Geometry check sheet. Reference: drawing and pictorial views, mm from the part's lowest x, y, z. A direction names the side the tool comes from. Round coordinates to 2 decimals unless told otherwise and drop trailing zeros. Loops run counter-clockwise (first coordinate to the right, second up) from the corner with the lowest first, then second, coordinate; pieces in that order, holes last. Notation, with made-up numbers: (46.25, 82.5) -> (58.25, 82.5) arc R12 ccw to (58.25, 101.5) -> close; hole circle Ø11 at (61.25, -7.75). An arc over 180 degrees is marked (long way). Use one line per item in the form item = value.
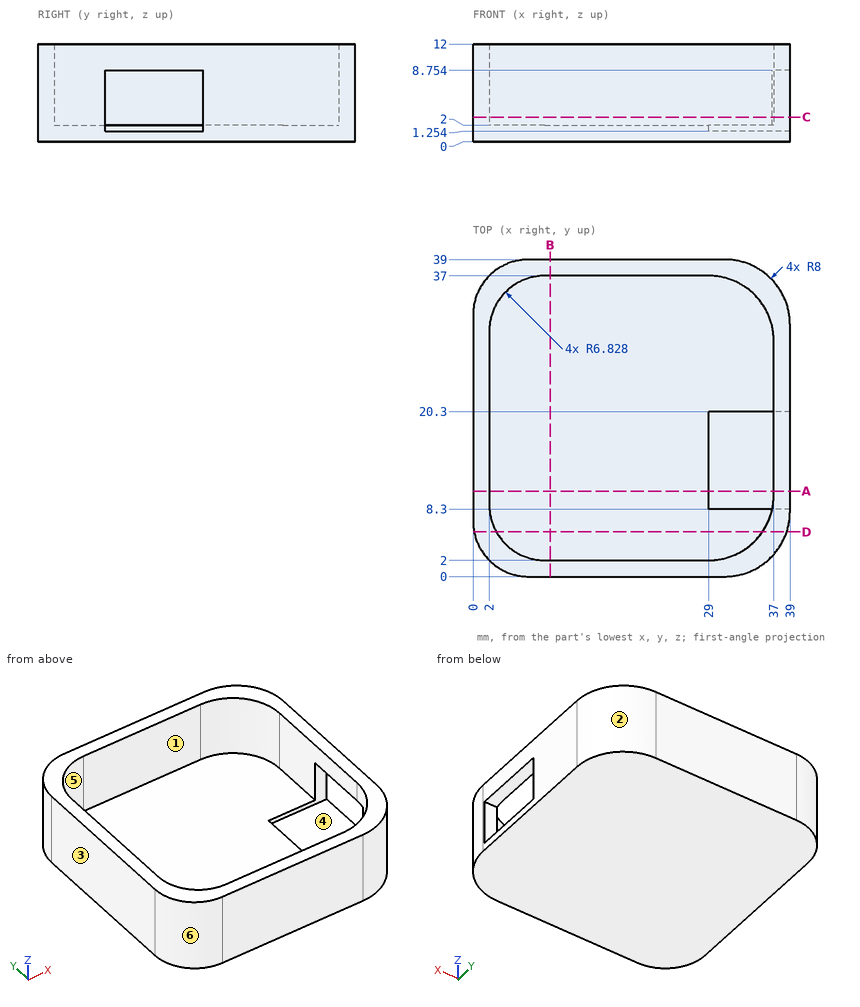
1. Material ranges on line 1 along X through (y, z) = (18.5, 11); line 2 along Z through (x, y) = (35.5, 21), recorded low to high.
Return value:
line_1 = 0 to 2, 37 to 39
line_2 = 0 to 2
2. Section check D-D (y = 5.5). Record the boundary of the cut face in (x, z), then the cut area to 3 significant figures.
Return value:
outline = (0.13, 0) -> (38.6, 0) -> (38.6, 12) -> (35.61, 12) -> (35.61, 2) -> (2.87, 2) -> (2.87, 12) -> (0.13, 12) -> close
area = 134 mm2
3. Section check C-C (z = 3). Record the boundary of the cut face in (x, y).
Return value:
outline = (0, 6.83) arc R6.83 ccw to (6.83, 0) -> (31, 0) arc R8 ccw to (39, 8) -> (39, 8.3) -> (36.82, 8.3) arc R8 cw to (29, 2) -> (8.83, 2) arc R6.83 cw to (2, 8.83) -> (2, 30.17) arc R6.83 cw to (8.83, 37) -> (29, 37) arc R8 cw to (37, 29) -> (37, 20.3) -> (39, 20.3) -> (39, 31) arc R8 ccw to (31, 39) -> (6.83, 39) arc R6.83 ccw to (0, 32.17) -> close
4. Gauge pin test, flat ends, axial feed: pin 1 (4 mm diameter, centred on x = 34.5, z = 6.5, fed in from +Y); pin 2 (3 mm diameter, centred on x = 21.5, y = 21.5, fed in from +Z). Record the tip position at first contact, or that the pin passes through.
Return value:
pin_1 = 38.86
pin_2 = 2
5. Tool access check on the marked faces 5 and 6. Record the directions out of +Z, -Z, +X, -X, +Y, -Y that give a thin tool (end or side, any length) a straight path to the whole face; none if there is none.
Return value:
face_5 = +Z
face_6 = +Z, -Z, -X, -Y
6. Section check A-A (y = 10.5). Record the boundary of the cut face in (x, z), then the cut area to 3 significant figures.
Return value:
outline = (0, 0) -> (39, 0) -> (39, 1.25) -> (29, 1.25) -> (29, 2) -> (2, 2) -> (2, 12) -> (0, 12) -> close; (37, 8.75) -> (39, 8.75) -> (39, 12) -> (37, 12) -> close
area = 97.0 mm2
7. Mould release check, pull along X, two halves, no side actions. Record for the marked faces 1, 2, 3 and 4: released by +X, released by -X, zero draft, split by the parting line, or undercut.
Return value:
face_1 = undercut
face_2 = released by +X
face_3 = released by -X
face_4 = zero draft
8. Section check B-B (x = 9.5). Record the boundary of the cut face in (y, z), then the cut area to 3 significant figures.
Return value:
outline = (0, 0) -> (39, 0) -> (39, 12) -> (37, 12) -> (37, 2) -> (2, 2) -> (2, 12) -> (0, 12) -> close
area = 118 mm2
